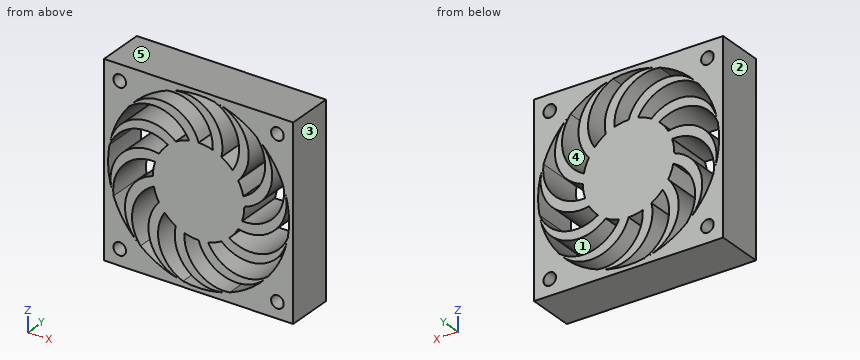
```python
from build123d import *

# Parameters (mm, degrees)
SKETCH1_W           = 60
SKETCH1_H           = 60
BOSS_EXTRUDE1_DEPTH = 15
SKETCH2_R           = 28.7
SKETCH2_R_2         = 14.5
CUT_EXTRUDE1_DEPTH  = 87.168439698
BOSS_EXTRUDE2_DEPTH = 15
CIRPATTERN1_COUNT   = 12
SKETCH4_R           = 2
CUT_EXTRUDE2_DEPTH  = 87.168439698


with BuildPart() as part:
    # Sketch1 → Boss-Extrude1 (new body)
    with BuildSketch(Plane(origin=(0, 0, 0), x_dir=(1, 0, 0), z_dir=(0, 1, 0))):
        with Locations((30, 30)):
            Rectangle(SKETCH1_W, SKETCH1_H)
    extrude(amount=BOSS_EXTRUDE1_DEPTH)

    # Sketch2 → Cut-Extrude1 (cut, through all)
    with BuildSketch(Plane(origin=(0, 15, 0), x_dir=(1, 0, 0), z_dir=(0, 1, 0))):
        with Locations(Location((30, 30, 0), (0, 0, 270))):
            Circle(SKETCH2_R)
        with Locations(Location((30, 30, 0), (0, 0, 270))):
            Circle(SKETCH2_R_2, mode=Mode.SUBTRACT)
    extrude(amount=-CUT_EXTRUDE1_DEPTH, mode=Mode.SUBTRACT)


with BuildPart() as cut_extrude1_piece_1:
    # of the separate pieces the step leaves, piece 1, a body of its own (cut_extrude1_pieces)
    add(part.part.solids().sort_by_distance((0, 0, 0))[0])



with BuildPart() as cut_extrude1_piece_2:
    # of the separate pieces the step leaves, piece 2, a body of its own (cut_extrude1_pieces)
    add(part.part.solids().sort_by_distance((30, 0, -15.5))[0])


with BuildPart() as cut_extrude1_piece_1_1:
    add(cut_extrude1_piece_1.part)

    add(cut_extrude1_piece_2.part)  # Boss-Extrude2 merges Cut-Extrude1 piece 2
    # Sketch3 → Boss-Extrude2 (add)
    with BuildSketch(Plane(origin=(0, 15, 0), x_dir=(1, 0, 0), z_dir=(0, 1, 0))):
        with BuildLine():
            ThreePointArc((30, 44.5), (39.309158475, 53.057700875), (51.346185748, 49.184117233))
            ThreePointArc((51.346185748, 49.184117233), (51.677164158, 48.809320936), (52.001562784, 48.428815346))
            ThreePointArc((52.001562784, 48.428815346), (41.493720217, 50.817966163), (33, 44.186260959))
            ThreePointArc((33, 44.186260959), (31.508180376, 44.421351946), (30, 44.5))
        make_face()
    boss_extrude2 = extrude(amount=-BOSS_EXTRUDE2_DEPTH)

    # CirPattern1: Boss-Extrude2 ×12 about axis
    cirpattern1_axis = Axis((30, 0, -30), (0, 1, 0))
    for i in range(1, CIRPATTERN1_COUNT):
        add(boss_extrude2.rotate(cirpattern1_axis, i * 360 / CIRPATTERN1_COUNT))

    # Sketch4 → Cut-Extrude2 (cut, through all)
    with BuildSketch(Plane(origin=(0, 15, 0), x_dir=(1, 0, 0), z_dir=(0, 1, 0))):
        with Locations(Location((5, 55, 0), (0, 0, 270))):
            Circle(SKETCH4_R)
        with Locations(Location((55, 55, 0), (0, 0, 270))):
            Circle(SKETCH4_R)
        with Locations(Location((55, 5, 0), (0, 0, 270))):
            Circle(SKETCH4_R)
        with Locations(Location((5, 5, 0), (0, 0, 270))):
            Circle(SKETCH4_R)
    extrude(amount=-CUT_EXTRUDE2_DEPTH, mode=Mode.SUBTRACT)


solid = cut_extrude1_piece_1_1.part
```
Can you work these out from the model? Positions are in its coordinate system, mm. Face numbers are marked on the shaded views. A direction names the side the tool comes from. Round coordinates to 2 decimals unless told otherwise and drop trailing zeros. Loops run counter-clockwise (first coordinate to the right, second up) from the corner with the lowest first, then second, coordinate; pieces in that order, holes last. Notation, with made-up numbers: M 52.5,-31.5 L 107.5,-31.5 A5 cw 107.5,-22.5 Z; hole C 70.5,-8.5 d10. An arc over 180 degrees is marked long. Write item = value, one per line. Start each with the question number.
(1) Which directions (+Z, -Z, +X, -X, +Y, -Y) give clear straight access to the entire face, cutting with the end or side of a thin tool? Please do the marked faces 4 and 5.
(2) Suppose I cut it at A-A on z = -5. Write out the boundary of the cut face in (x, y), plus the area to 3 significant figures.
(3) I need wall thicknesses on line 1 along X through (y, z) = (8, -5); line 2 along Z through (x, y) = (4.5, 14.25); line 3 along X through (y, z) = (4.5, -12.5). Which ranges of each line are inside material? Lowest first, please.
(4) Suppose I cut it at D-D on x = 5. Write out the boundary of the cut face in (y, z).
(5) If we mould it in two halves opening along X, with no side actions, what happens to the marked faces 1, 2 and 3? For each: released by +X, released by -X, zero draft, split by the parting line, or undercut.
(6) Suppose I cut it at B-B on x = 29. Write out the boundary of the cut face in (y, z).
(7) Suppose I cut it at C-C on y = 2.5. Give the number of separate pieces and of enclosed holes in the cut face, plus the area to 3 significant figures.
(8) I'm going to push a flat-ended pin straight in: P1, Ø2.5, axis at x = 55, z = -55, coming from the -Y side. Where does the tip first touch, or does it pass through?
Answer block:
q1.face_4 = +Y, -Y
q1.face_5 = +Z, +X, -X, +Y, -Y
q2.outline = M 0,0 L 3,0 L 3,15 L 0,15 Z; M 7,0 L 15.9,0 L 15.9,15 L 7,15 Z; M 28.89,0 L 33.03,0 L 33.03,15 L 28.89,15 Z; M 39.64,0 L 41.88,0 L 41.88,15 L 39.64,15 Z; M 44.1,0 L 53,0 L 53,15 L 44.1,15 Z; M 57,0 L 60,0 L 60,15 L 57,15 Z
q2.area = 453 mm²
q3.line_1 = 0 to 3, 7 to 15.9, 28.89 to 33.03, 39.64 to 41.88, 44.1 to 53, 57 to 60
q3.line_2 = -60 to -56.94, -53.06 to -43.17, -31.93 to -27.61, -20.84 to -18.69, -16.83 to -6.94, -3.06 to 0
q3.line_3 = 0 to 7.25, 24.59 to 28.62, 34.16 to 37.38, 42.83 to 45.79, 50.69 to 52.08, 52.75 to 60
q4.outline = M 0,-60 L 15,-60 L 15,-57 L 0,-57 Z; M 0,-53 L 15,-53 L 15,-44.1 L 0,-44.1 Z; M 0,-31.11 L 15,-31.11 L 15,-26.97 L 0,-26.97 Z; M 0,-20.36 L 15,-20.36 L 15,-18.12 L 0,-18.12 Z; M 0,-15.9 L 15,-15.9 L 15,-7 L 0,-7 Z; M 0,-3 L 15,-3 L 15,0 L 0,0 Z
q5.face_1 = undercut
q5.face_2 = released by -X
q5.face_3 = released by +X
q6.outline = M 0,-60 L 15,-60 L 15,-58.68 L 0,-58.68 Z; M 0,-56.38 L 15,-56.38 L 15,-53.24 L 0,-53.24 Z; M 0,-44.47 L 15,-44.47 L 15,-13.15 L 0,-13.15 Z; M 0,-5.07 L 15,-5.07 L 15,-2.75 L 0,-2.75 Z; M 0,-1.32 L 15,-1.32 L 15,0 L 0,0 Z
q7.separate_pieces = 1
q7.enclosed_holes = 16
q7.area = 2,280 mm²
q8.P1 = through
